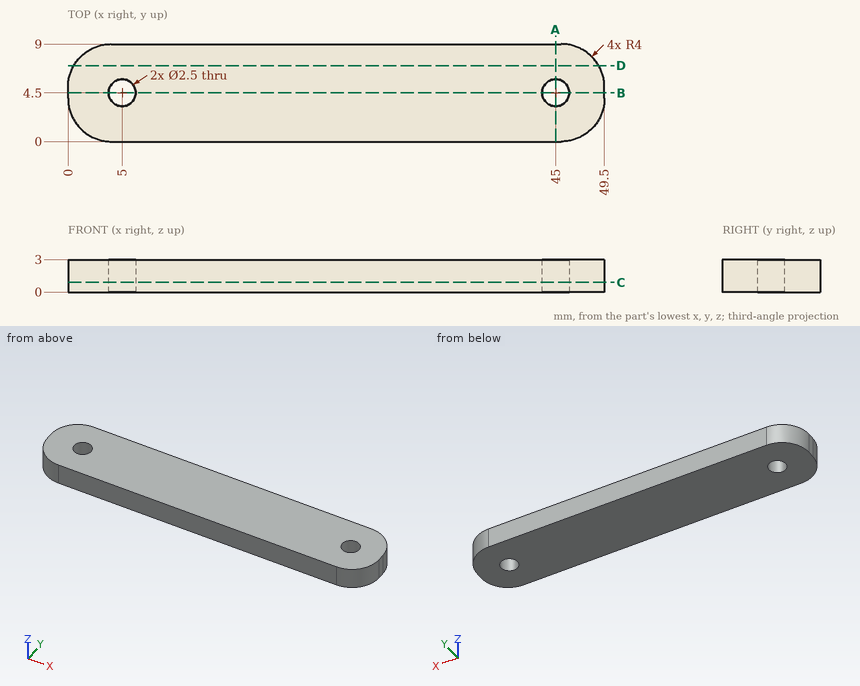
Study the drawing (mm; zero at the part's minimum x, y, z) and answer. Give positions to 0.01 mm unless a question says otherwise; leave off trailing zeros. Loops run counter-clockwise (first coordinate to the right, second up) from the corner with the lowest first, then second, coordinate; pieces in that order, holes last. Notation, with made-up numbers: M 8,49.25 L 60,49.25 A33 ccw 60,86.25 Z; hole C -22,-21.75 d4. An arc over 180 degrees is marked long. One line per item, written item: value.
1. Find the intervals of material crossed by probe 1 along Y at (x, z) = (5, 1.15); probe 2 along X at (y, z) = (5.5, 0.8); probe 3 along X at (y, z) = (4.75, 0.75), in increasing order.
Found:
probe 1: 0 to 3.25, 5.75 to 9
probe 2: 0.03 to 4.25, 5.75 to 44.25, 45.75 to 49.47
probe 3: 0 to 3.78, 6.22 to 43.78, 46.22 to 49.5
2. Section C-C on z = 0.9 is taken. Determine the outline of the cut face in (x, y).
Found:
outline: M 0,4 A4 ccw 4,0 L 45.5,0 A4 ccw 49.5,4 L 49.5,5 A4 ccw 45.5,9 L 4,9 A4 ccw 0,5 Z; hole C 5,4.5 d2.5; hole C 45,4.5 d2.5
3. Section B-B on y = 4.5 is taken. Determine the outline of the cut face in (x, z), plus the area to 4 significant figures.
Found:
outline: M 0,0 L 3.75,0 L 3.75,3 L 0,3 Z; M 6.25,0 L 43.75,0 L 43.75,3 L 6.25,3 Z; M 46.25,0 L 49.5,0 L 49.5,3 L 46.25,3 Z
area: 133.5 mm^2
4. Section D-D on y = 7 is taken. Determine the outline of the cut face in (x, z).
Found:
outline: M 0.54,0 L 48.96,0 L 48.96,3 L 0.54,3 Z
5. Each of these flat-tipped pins is pushed along its axis until it touches: P1, Ø3, axis at x = 22, y = 1, coming from the -Z side; P2, Ø2, axis at x = 5, y = 4.5, coming from the -Z side. Where does it stop, or does it pass through?
Found:
P1: z = 0
P2: through
6. Section A-A on x = 45 is taken. Determine the outline of the cut face in (y, z).
Found:
outline: M 0,0 L 3.25,0 L 3.25,3 L 0,3 Z; M 5.75,0 L 9,0 L 9,3 L 5.75,3 Z
